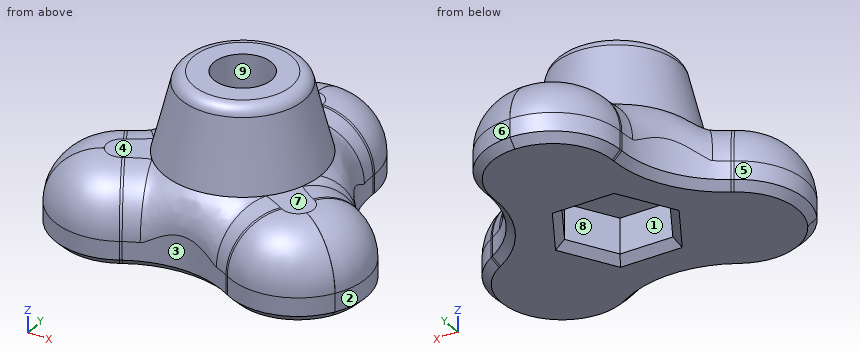
from build123d import *

# Parameters (mm, degrees)
PAD_DEPTH       = 6
FILLET_R        = 8
FILLET001_R     = 5.19
FILLET002_R     = 4
SKETCH002_R     = 2.2
POCKET_DEPTH    = 12.001
POCKET001_DEPTH = 3.3
SKETCH005_R     = 2.2
PAD001_DEPTH    = 0.3
FILLET003_R     = 1
CHAMFER_SIZE    = 0.6
CHAMFER001_SIZE = 0.6


with BuildPart() as revolution:
    # Sketch004 → Revolution (revolve)
    with BuildSketch(Plane.XZ):
        Polygon((4.5, 12), (0, 12), (0, 6), (6, 6), align=None)
    revolve(axis=Axis((0, 0, 0), (0, 0, 1)))


with BuildPart() as chamfer001:
    # Sketch → Pad (new body)
    with BuildSketch(Plane.XY):
        Polygon((-5.196152, 3), (-5.196152, 13), (5.196152, 13), (5.196152, 3), (13.856406, -2), (8.660254, -11), (0, -6), (-8.660254, -11), (-13.856406, -2), align=None)
    extrude(amount=PAD_DEPTH)

    # Fillet
    fillet_edges = [chamfer001.edges().sort_by_distance(p)[0] for p in [
        (-5.196152, 3, 3),
        (5.196152, 3, 3),
        (0, -6, 3),
    ]]
    fillet(fillet_edges, radius=FILLET_R)

    # Fusion: union Revolution
    add(revolution.part)

    # Fillet001
    fillet001_edges = [chamfer001.edges().sort_by_distance(p)[0] for p in [
        (-8.660254, -11, 3),
        (-13.856406, -2, 3),
        (-5.196152, 13, 3),
        (5.196152, 13, 3),
        (13.856406, -2, 3),
        (8.660254, -11, 3),
    ]]
    fillet(fillet001_edges, radius=FILLET001_R)

    # Fillet002
    fillet002_edges = [chamfer001.edges().sort_by_distance(p)[0] for p in [
        (6.267949, 3.618802, 6),
    ]]
    fillet(fillet002_edges, radius=FILLET002_R)

    # Sketch002 → Pocket (cut, through all)
    with BuildSketch(Plane.XY.offset(12)):
        Circle(SKETCH002_R)
    extrude(amount=-POCKET_DEPTH, mode=Mode.SUBTRACT)

    # Sketch003 → Pocket001 (cut)
    with BuildSketch(Plane(origin=(0, 0, 0), x_dir=(1, 0, 0), z_dir=(0, 0, -1))):
        Polygon((4.070319, 0), (2.03516, 3.525), (-2.03516, 3.525), (-4.070319, 0), (-2.03516, -3.525), (2.03516, -3.525), align=None)
    extrude(amount=-POCKET001_DEPTH, mode=Mode.SUBTRACT)

    # Sketch005 → Pad001 (new body)
    with BuildSketch(Plane(origin=(0, 0, 3.3), x_dir=(1, 0, 0), z_dir=(0, 0, -1))):
        Circle(SKETCH005_R)
    extrude(amount=-PAD001_DEPTH)

    # Fillet003
    fillet003_edges = [chamfer001.edges().sort_by_distance(p)[0] for p in [
        (-4.5, 0, 12),
    ]]
    fillet(fillet003_edges, radius=FILLET003_R)

    # Chamfer
    chamfer_edges = [chamfer001.edges().sort_by_distance(p)[0] for p in [
        (-6.267949, 3.618802, 0),
    ]]
    chamfer(chamfer_edges, length=CHAMFER_SIZE)

    # Chamfer001
    chamfer001_edges = [chamfer001.edges().sort_by_distance(p)[0] for p in [
        (3.05274, 1.7625, 0),
        (0, 3.525, 0),
        (-3.05274, 1.7625, 0),
        (-3.05274, -1.7625, 0),
        (0, -3.525, 0),
        (3.05274, -1.7625, 0),
    ]]
    chamfer(chamfer001_edges, length=CHAMFER001_SIZE)


solid = chamfer001.part
CAD build for the part. Positions are in the model's coordinates, mm. Face numbers are marked on the shaded views. A direction names the side the tool comes from. Round coordinates to 2 decimals unless told otherwise and drop trailing zeros. Order: outer loops, then holes, each group sorted by start corner. A loop starts at its lowest first (then second) coordinate and runs counter-clockwise, first axis right, second up. Notation, with made-up numbers: (88, 25.25) - (120, 25.25) arc R24 ccw to (120, 47.25) - close; hole circle Ø5 at (56, -34). An arc over 180 degrees is marked (long way). Return JSON: item names as keys, results as strings.
(1) Cut at C-C (z = 6.5). Give the cut face in (x, y) (3 decimals), then the cut area to 3 significant figures.
Answer key:
{"outline": "circle Ø11.75 at (0, 0); hole circle Ø4.4 at (0, 0)", "area": "93.2 mm^2"}
(2) Tool access for the marked faces 5, 6, 7, 8 and 9: list every direction of +Z, -Z, +X, -X, +Y, -Y with a clear straight run to the whole face (end or side of a thin tool).
Answer key:
{"face 5": "+Z, -Z, -X", "face 6": "+Z, -Z, +X, +Y", "face 7": "+Z, +X, -Y", "face 8": "-Z", "face 9": "+Z"}
(3) Pull direction Y, two halves, no side cores. Call the marked faces 1, 2, 3 and 4: +Y half, -Y half, draft (parallel to the pull), parting line (faces both ways), or undercut.
Answer key:
{"face 1": "undercut", "face 2": "parting line", "face 3": "-Y half", "face 4": "draft"}
(4) Pin check, flat tips, straight feed: pin 1 Ø12 at (x, y) = (-9, 5.5) entering from +Z; pin 2 Ø0.8 at (x, y) = (0, 8) entering from +Z; pin 3 Ø3.5 at (x, y) = (-0.5, 1.5) entering from -Z. Stop position of each tip, or through.
Answer key:
{"pin 1": "stops at z = 11.56", "pin 2": "stops at z = 6", "pin 3": "stops at z = 3.3"}
(5) Cut at B-B (z = 8). Give the cut face in (x, y).
Answer key:
{"outline": "circle Ø11 at (0, 0); hole circle Ø4.4 at (0, 0)"}
(6) Cut at A-A (z = 1.5). Give the cut face in (x, y) (3 decimals).
Answer key:
{"outline": "(-11.261, -6.495) - (-11.255, -6.505) arc R5.19 ccw to (-4.166, -8.405) - (-4, -8.309) arc R8 cw to (4, -8.309) - (4.166, -8.405) arc R5.19 ccw to (11.255, -6.505) - (11.261, -6.495) arc R5.19 ccw to (9.362, 0.595) - (9.196, 0.691) arc R8 cw to (5.196, 7.619) - (5.196, 7.81) arc R5.19 ccw to (0.006, 13) - (-0.006, 13) arc R5.19 ccw to (-5.196, 7.81) - (-5.196, 7.619) arc R8 cw to (-9.196, 0.691) - (-9.362, 0.595) arc R5.19 ccw to start; hole (-4.07, 0) - (-2.035, -3.525) - (2.035, -3.525) - (4.07, 0) - (2.035, 3.525) - (-2.035, 3.525) - close"}
(7) Wall check: probe 1 along X at (y, z) = (0.5, 2); probe 2 along X at (y, z) = (0.5, 3); probe 3 along Z at (x, y) = (-6.25, -5.25). Give the ranges that are in metal, low to high. Write a range as from..to.
Answer key:
{"probe 1": "x = -9.52..-3.78, 3.78..9.52", "probe 2": "x = -9.27..-3.78, 3.78..9.27", "probe 3": "z = 0..5.99"}
